Autodesk Inventor part; units mm, degrees
ref_plane "YZ Plane" through (0, 0, 0) normal (1, 0, 0) x (0, 1, 0)
ref_plane "XZ Plane" through (0, 0, 0) normal (0, 1, 0) x (-1, 0, 0)
ref_plane "XY Plane" through (0, 0, 0) normal (0, 0, 1) x (1, 0, 0)
sketch "スケッチ1" plane through (0, 0, 0) normal (0, 0, 1) x (1, 0, 0)
  circle A0 centre (0, 0) radius 4
  dimension "d0" = 8
extrude "押し出し1" add sketch "スケッチ1" along normal blind 142
sketch "スケッチ2" plane through (0, 0, 142) normal (0, 0, 1) x (1, 0, 0)
  circle A0 centre (0, 0) radius 2
  dimension "d3" = 4
extrude "押し出し2" cut sketch "スケッチ2" against normal blind 10
sketch "スケッチ3" plane through (0, 0, 0) normal (0, 0, -1) x (-1, 0, 0)
  circle A0 centre (0, 0) radius 2
  dimension "d6" = 4
extrude "押し出し3" cut sketch "スケッチ3" against normal blind 10
thread "ねじ1"
thread "ねじ2"
properties part number "シャフト" material "ポリカーボネート、スモーク"
Design review of the part built by this model. Coordinates are the model's own, in mm. A direction names the side the tool comes from. Coordinates: 2 decimals unless noted, no trailing zeros. Loops run counter-clockwise (first coordinate to the right, second up) from the corner with the lowest first, then second, coordinate; pieces in that order, holes last. Notation, with made-up numbers: M 19.5,-11.5 L 50.5,-11.5 A19 ccw 50.5,13.5 Z; hole C 0,2.5 d4. An arc over 180 degrees is marked long. Use one line per item in the form item = value.
(1) For line 1 along Y through (x, z) = (0, 139); line 2 along Z through (x, y) = (-1.75, 0); line 3 along X through (y, z) = (-1.5, 126), list the stretches that pass through material, from the lowest coordinate up. Write a range as from..to.
Return value:
line_1 = -4..-2, 2..4
line_2 = 10..132
line_3 = -3.71..3.71
(2) Clearance check with flat-ended pins moving along their axes: P1, Ø3.5, axis at x = 0, y = 0, coming from the -Z side; P2, Ø3.5, axis at x = 0, y = 0, coming from the +Z side; P3, Ø4, axis at y = 2.5, z = 44.5, coming from the -X side. State where each tip first meets the part, or that it passes through.
Return value:
P1 = 10
P2 = 132
P3 = -3.97
(3) Consider section C-C (z = 107.5). Write out the cut boundary in (x, y).
Return value:
outline = C 0,0 d8
(4) Draft analysis for pull direction Y (two halves, no side actions). For faces 1 (the face through (0, -2, 5)), 2 (the face through (0, 0, 132)), 3 (the face through (-0.867, 3.905, 70.006)), 4 (the face through (-2, -1, 0)), state which applies: pulls with the +Y half, pulls with the -Y half, needs draft (parallel to the pull), parting line crosses it, or undercut.
Return value:
face_1 = undercut
face_2 = undercut
face_3 = parting line crosses it
face_4 = needs draft
(5) For faces 5 (the face through (-2, -1, 142)), 6 (the face through (0, 0, 10)), 7 (the face through (0, -2, 137)), list the 3-axis set-ups (+Z, -Z, +X, -X, +Y, -Y) from which the entire face can be reached by the end or side of a thin tool; tool diameter is ignored.
Return value:
face_5 = +Z, +X, -X, +Y, -Y
face_6 = -Z
face_7 = +Z
(6) Consider section A-A (y = 0). Write out the cut boundary in (x, z), and give its area (3 significant figures).
Return value:
outline = M -4,0 L -2,0 L -2,10 L 2,10 L 2,0 L 4,0 L 4,142 L 2,142 L 2,132 L -2,132 L -2,142 L -4,142 Z
area = 1,060 mm2
